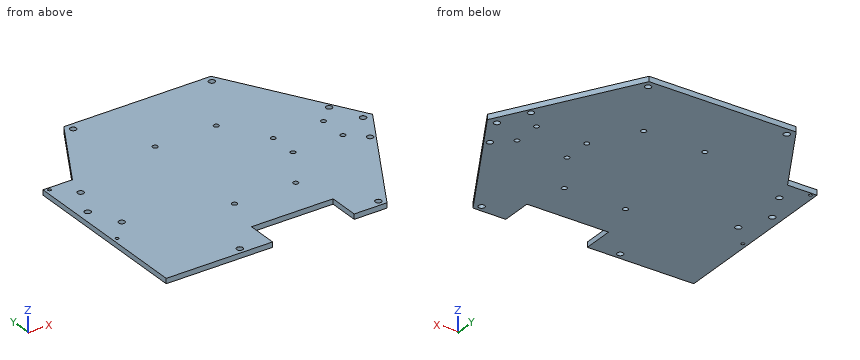
from build123d import *

# Parameters (mm, degrees)
EXTRUDE_3_DEPTH                 = 5
HOLE_WIZARD_6_0_6_1_D           = 6
HOLE_WIZARD_6_0_6_1_CSINK_D     = 6.05
HOLE_WIZARD_6_0_6_1_CSINK_ANGLE = 90
SKETCH_20_R                     = 2.4
CUT_EXTRUDE_2_DEPTH             = 192.006108105
SKETCH_33_R                     = 3
CUT_EXTRUDE_3_DEPTH             = 192.006108105
SKETCH_34_R                     = 2.5
CUT_EXTRUDE_4_DEPTH             = 192.006108105
SKETCH_35_R                     = 1.6
EXTRUDE_5_DEPTH                 = 5


with BuildPart() as part:
    # 草图8 → 凸台-拉伸3 (new body)
    with BuildSketch(Plane.XY):
        Polygon((144.337567297, 0), (72.168783649, 125), (-72.168783649, 125), (-144.337567297, 0), (-72.168783649, -125), (-40, -125), (-40, -95), (40, -95), (40, -125), (72.168783649, -125), align=None)
    extrude(amount=EXTRUDE_3_DEPTH)

    # Ø6.0 (6) 直径孔1 (through all)
    with Locations(Plane.XY.offset(5)):
        with Locations((-135.003092598, 0), (-67.980688817, -118.866778441), (-67.980688817, 117.662022204)):
            hole_wizard_6_0_6_1 = CounterSinkHole(HOLE_WIZARD_6_0_6_1_D / 2, HOLE_WIZARD_6_0_6_1_CSINK_D / 2, counter_sink_angle=HOLE_WIZARD_6_0_6_1_CSINK_ANGLE)

    # 镜向2: Ø6.0 (6) 直径孔1 across plane
    add(hole_wizard_6_0_6_1.mirror(Plane(origin=(0, 0, 0), x_dir=(0, 0, 1), z_dir=(1, 0, 0))), mode=Mode.SUBTRACT)

    # 草图20 → 切除-拉伸2 (cut, through all)
    with BuildSketch(Plane.XY.offset(5)):
        with Locations((56.370867728, 13.653021969)):
            Circle(SKETCH_20_R)
        with Locations((105.370867728, 13.324633606)):
            Circle(SKETCH_20_R)
        with Locations((56.370867728, -14.346978031)):
            Circle(SKETCH_20_R)
        with Locations((105.370867728, -14.346978031)):
            Circle(SKETCH_20_R)
    extrude(amount=-CUT_EXTRUDE_2_DEPTH, mode=Mode.SUBTRACT)

    # 草图33 → 切除-拉伸3 (cut, through all)
    with BuildSketch(Plane.XY.offset(5)):
        with Locations((-121.797773, -29.181235)):
            Circle(SKETCH_33_R)
        with Locations(Location((121.797773, -29.181235, 0), (0, 0, 180))):
            Circle(SKETCH_33_R)
        with Locations((121.797773, 29.181235)):
            Circle(SKETCH_33_R)
        with Locations(Location((-121.797773, 29.181235, 0), (0, 0, 180))):
            Circle(SKETCH_33_R)
    extrude(amount=-CUT_EXTRUDE_3_DEPTH, mode=Mode.SUBTRACT)

    # 草图34 → 切除-拉伸4 (cut, through all)
    with BuildSketch(Plane.XY.offset(5)):
        with Locations((-30, -56.392396)):
            Circle(SKETCH_34_R)
        with Locations(Location((30, -56.392396, 0), (0, 0, 180))):
            Circle(SKETCH_34_R)
        with Locations((30, 56.392396)):
            Circle(SKETCH_34_R)
        with Locations(Location((-30, 56.392396, 0), (0, 0, 180))):
            Circle(SKETCH_34_R)
    extrude(amount=-CUT_EXTRUDE_4_DEPTH, mode=Mode.SUBTRACT)

    # 草图35 → 凸台-拉伸5 (add)
    # profile 1 of 2: a face of its own
    with BuildSketch(Plane.XY):
        Polygon((-144.337567297, 0), (-115.470053838, 50), (-144.337567297, 50), align=None)
        with Locations((-140, 47)):
            Circle(SKETCH_35_R, mode=Mode.SUBTRACT)
    # profile 2 of 2: a face of its own
    with BuildSketch(Plane.XY):
        Polygon((-72.168783649, -125), (-144.337567297, 0), (-144.337567297, -125), align=None)
        with Locations((-140, -49)):
            Circle(SKETCH_35_R, mode=Mode.SUBTRACT)
    extrude(amount=EXTRUDE_5_DEPTH)


solid = part.part
Read the model definition and answer for the solid it produces. Units are mm, in the model's axes. Coordinates: 2 decimals unless noted, no trailing zeros. Loops run counter-clockwise (first coordinate to the right, second up) from the corner with the lowest first, then second, coordinate; pieces in that order, holes last. Notation, with made-up numbers: (7, 22.25) -> (11, 22.25) arc R18 ccw to (11, 39.25) -> close; hole circle Ø8 at (25, 4). An arc over 180 degrees is marked (long way). Write item = value, one per line. Start each with the question number.
1) The part is cut by section B-B, the plane x = -90. Determine the outline of the cut face in (y, z).
2) The part is cut by section C-C, the plane y = -20. Determine the outline of the cut face in (x, z), plus the area to 3 significant figures.
3) Given P1, Ø2.5, axis at x = 10.5, z = 2, coming from the -Y side; P2, Ø1, axis at y = -87, z = 2, coming from the +X side, each flat-ended and moving along its own axis, determine where each tip first touches the part or whether it passes through.
4) The part is cut by section A-A, the plane z = 2.25. State how many separate pieces and enclosed holes the cut face has, plus the area to 3 significant figures.
5) Find the intervals of material crossed by L1, parallel to Y at x = -140, z = 2.9; L2, parallel to Y at x = -30, z = 3.7; L3, parallel to X at y = 0.5, z = 0.7, in increasing order. Write a range as from..to.
Result:
q1.outline = (-125, 0) -> (94.12, 0) -> (94.12, 5) -> (-125, 5) -> close
q2.outline = (-144.34, 0) -> (132.79, 0) -> (132.79, 5) -> (-144.34, 5) -> close
q2.area = 1,390 mm²
q3.P1 = -95
q3.P2 = 94.4
q4.separate_pieces = 1
q4.enclosed_holes = 20
q4.area = 56,500 mm²
q5.L1 = -125..-50.6, -47.4..45.4, 48.6..50
q5.L2 = -95..-58.89, -53.89..53.89, 58.89..125
q5.L3 = -144.34..-137.96, -132.05..132.05, 137.96..144.05
